Source: CAD feature listing. Evaluate the final solid. Frame: model axes, mm. Face numbers are marked on the shaded views. A direction names the side the tool comes from. Round coordinates to 2 decimals unless told otherwise and drop trailing zeros. Loops run counter-clockwise (first coordinate to the right, second up) from the corner with the lowest first, then second, coordinate; pieces in that order, holes last. Notation, with made-up numbers: (52, 51) -> (65, 51) arc R32 ccw to (65, 78) -> close; hole circle Ø7 at (-8, -15.75). An arc over 180 degrees is marked (long way). Put each result on its own line as item: value. Start each with the question number.
1. Set-up query: the marked faces 5 and 6. Return all of +Z, -Z, +X, -X, +Y, -Y with unobstructed straight access to the full face (end or side cutting, diameter ignored); none if empty.
2. Cut plane D-D (z = 2.75). Return the cut outline in (x, y) (3 decimals), then the cut area to 3 significant figures.
3. Draft query along Y for the marked faces 1, 2, 3 and 4. Return one class per face: pulls with the +Y half, pulls with the -Y half, needs draft (parallel to the pull), parting line crosses it, or undercut.
4. Cut plane C-C (x = -10). Return the cut outline in (y, z) (3 decimals), then the cut area to 3 significant figures.
5. Cut plane A-A (x = 10). Return the cut outline in (y, z) (3 decimals), then the cut area to 3 significant figures.
6. Cut plane B-B (z = 9.75). Return the cut outline in (x, y) (3 decimals).
7. Contact query for flat-ended pins moving along their axis: pin 1 (5 mm diameter, centred on y = -0.5, z = 5, fed in from +X); pin 2 (1 mm diameter, centred on y = 6, z = 10.5, fed in from -X); pin 3 (4 mm diameter, centred on y = -5, z = 8.5, fed in from +X); pin 4 (5 mm diameter, centred on x = 6.5, y = 1.5, fed in from +Z). Output: stop coordinate, or through.
8. Material intervals for L1, parallel to Y at x = 10, z = 10.3 (3 decimals); L2, parallel to Z at x = 8, y = 6.5; L3, parallel to X at y = 5.5, z = 1, sorted ascending.
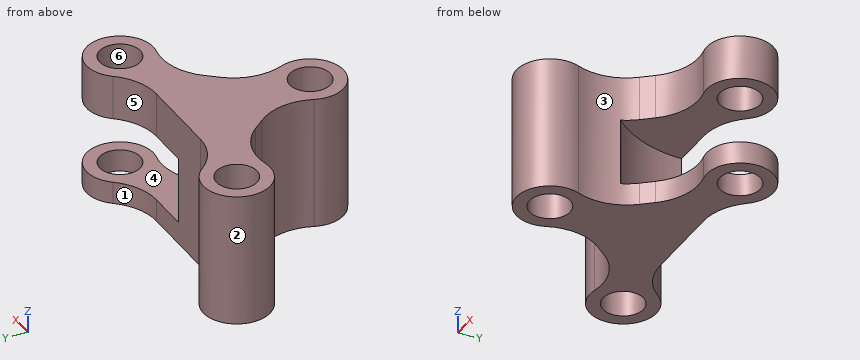
```python
from build123d import *

# Parameters (mm, degrees)
ESQUISSE2_R             = 3
ESQUISSE2_R_2           = 1.825
BOSS_EXTRU_1_DEPTH      = 12
ESQUISSE3_R             = 10
ENL_V_MAT_EXTRU_1_DEPTH = 6
CONG_1_R                = 5
FILLET1_R               = 5


with BuildPart() as part:
    # Esquisse2 → Boss.-Extru.1 (new body)
    # profile 1 of 4: a face of its own
    with BuildSketch(Plane.XY):
        with Locations((-10, 5)):
            Circle(ESQUISSE2_R)
        with Locations((-10, 5)):
            Circle(ESQUISSE2_R_2, mode=Mode.SUBTRACT)
    # profile 2 of 4: a face of its own
    with BuildSketch(Plane.XY):
        with Locations((10, 5)):
            Circle(ESQUISSE2_R)
        with Locations((10, 5)):
            Circle(ESQUISSE2_R_2, mode=Mode.SUBTRACT)
    # profile 3 of 4: a face of its own
    with BuildSketch(Plane.XY):
        with Locations((0, -6.825)):
            Circle(ESQUISSE2_R)
        with Locations((0, -6.825)):
            Circle(ESQUISSE2_R_2, mode=Mode.SUBTRACT)
    # profile 4 of 4: a face of its own
    with BuildSketch(Plane.XY):
        Polygon((-8.175, 5), (8.175, 5), (0, -5), align=None)
    extrude(amount=BOSS_EXTRU_1_DEPTH)

    # Esquisse3 → Enlèv. mat.-Extru.1 (cut)
    with BuildSketch(Plane.XY.offset(2)):
        with Locations((10, 5)):
            Circle(ESQUISSE3_R)
    extrude(amount=ENL_V_MAT_EXTRU_1_DEPTH, mode=Mode.SUBTRACT)

    # Congé1
    # the kernel refuses this fillet: 5 mm, written as the material it adds along each edge
    with BuildSketch(Plane(origin=(-7, 5, 0), x_dir=(-0.3311912213512006, 0.9435636570469954, 0), z_dir=(0, 0, 1))) as cong_1_piece_1:
        with BuildLine():
            CenterArc((3.643103435, -4.717818285), CONG_1_R, 109.341093727, 51.317812547)
            Line((-1.07471485, -3.061862178), (0, 0))
            ThreePointArc((0, 0), (0.993573664, -0.169309029), (1.987147328, 0))
        make_face()
    extrude(amount=12)
    with BuildSketch(Plane(origin=(-7.231093941, 3.845374851, 12), x_dir=(-0.7661000074497634, -0.6427213848826507, 0), z_dir=(0, 0, -1))) as cong_1_piece_2:
        with BuildLine():
            CenterArc((5.056907819, -4.440322454), CONG_1_R, 117.368969646, 63.360078756)
            Line((0.057312583, -4.503942212), (0, 0))
            ThreePointArc((0, 0), (1.379156678, -0.335806528), (2.758313356, 0))
        make_face()
    extrude(amount=12)
    with BuildSketch(Plane(origin=(-0.858096974, -3.950340093, 12), x_dir=(-0.6329215353519139, 0.7742159453846039, 0), z_dir=(0, 0, -1))) as cong_1_piece_3:
        with BuildLine():
            CenterArc((4.246739065, -5), CONG_1_R, 90, 61.27443838)
            ThreePointArc((-0.137920096, -2.596926126), (0.227062491, -1.314184518), (0, 0))
            Line((0, 0), (4.246739065, 0))
        make_face()
    extrude(amount=12)
    with BuildSketch(Plane(origin=(7.231093941, 3.845374851, 12), x_dir=(-0.6329215353519138, -0.774215945384604, 0), z_dir=(0, 0, -1))) as cong_1_piece_4:
        with BuildLine():
            CenterArc((4.504306848, -5), CONG_1_R, 90, 63.360078756)
            ThreePointArc((0.035096646, -2.758090063), (0.353327666, -1.374772245), (0, 0))
            Line((0, 0), (4.504306848, 0))
        make_face()
    extrude(amount=4)
    with BuildSketch(Plane(origin=(7, 5, 12), x_dir=(-1, 0, 0), z_dir=(0, 0, -1))) as cong_1_piece_5:
        with BuildLine():
            CenterArc((3.244997998, 5), CONG_1_R, 218.682187453, 51.317812547)
            ThreePointArc((-0.658125751, 1.875), (-0.169309029, 0.993573664), (0, 0))
            Line((0, 0), (3.244997998, 0))
        make_face()
    extrude(amount=4)
    with BuildSketch(Plane(origin=(0.858096974, -3.950340093, 12), x_dir=(0.7395598752725667, -0.6730907746261462, 0), z_dir=(0, 0, -1))) as cong_1_piece_6_section:
        with BuildLine():
            CenterArc((4.767740899, -4.505933799), CONG_1_R, 115.685497342, 61.27443838)
            Line((-0.225222573, -4.240762606), (0, 0))
            ThreePointArc((0, 0), (1.300292973, -0.29643972), (2.600585945, 0))
        make_face()
    cong_1_piece_6 = extrude(amount=12, mode=Mode.PRIVATE)
    cong_1_piece_6 = cong_1_piece_6 - Plane(origin=(10, 5, 10), x_dir=(1, 0, 0), z_dir=(0, 0, -1)) * Cylinder(10, 41, mode=Mode.PRIVATE)
    add(cong_1_piece_6)
    with BuildSketch(Plane(origin=(0.858096974, -3.950340093, 12), x_dir=(0.7395598752725667, -0.6730907746261462, 0), z_dir=(0, 0, -1))) as cong_1_piece_7_section:
        with BuildLine():
            CenterArc((4.767740899, -4.505933799), CONG_1_R, 115.685497342, 61.27443838)
            Line((-0.225222573, -4.240762606), (0, 0))
            ThreePointArc((0, 0), (1.300292973, -0.29643972), (2.600585945, 0))
        make_face()
    cong_1_piece_7 = extrude(amount=22.616847663, mode=Mode.PRIVATE)
    cong_1_piece_7 = split(cong_1_piece_7, bisect_by=Plane(origin=(2.909028405, -1.544063306, 8), z_dir=(0, 0, 1)), keep=Keep.TOP, mode=Mode.PRIVATE)
    add(cong_1_piece_7)
    with BuildSketch(Plane(origin=(0.858096974, -3.950340093, 22.616847663), x_dir=(0.7395598752725666, -0.6730907746261463, 0), z_dir=(0, 0, -1))) as cong_1_piece_8_section:
        with BuildLine():
            CenterArc((4.767740899, -4.505933799), CONG_1_R, 115.685497342, 61.27443838)
            Line((-0.225222573, -4.240762606), (0, 0))
            ThreePointArc((0, 0), (1.300292973, -0.29643972), (2.600585945, 0))
        make_face()
    cong_1_piece_8 = extrude(amount=22.616847663, mode=Mode.PRIVATE)
    cong_1_piece_8 = split(cong_1_piece_8, bisect_by=Plane(origin=(2.909028405, -1.544063306, 2), z_dir=(0, 0, -1)), keep=Keep.TOP, mode=Mode.PRIVATE)
    add(cong_1_piece_8)

    # Fillet1
    fillet1_edges = [part.edges().sort_by_distance(p)[0] for p in [
        (7.231093941, 3.845374851, 1),
        (7, 5, 1),
    ]]
    fillet(fillet1_edges, radius=FILLET1_R)


solid = part.part
```
Solution:
1. face 5: +Z, -Z, +Y
1. face 6: +Z, -Z
2. outline: (-9.344, 2.073) arc R5 cw to (-4.38, 0.358) -> (-3.546, -0.662) arc R5 cw to (-2.781, -5.701) arc R3 ccw (long way) to (2.781, -5.701) arc R5 cw to (2.791, -1.93) arc R10 cw to (0, 5) -> (-3.755, 5) arc R5 cw to (-7.658, 6.875) arc R3 ccw (long way) to start; hole circle Ø3.65 at (-10, 5); hole circle Ø3.65 at (0, -6.825)
2. area: 94.0 mm^2
3. face 1: pulls with the +Y half
3. face 2: parting line crosses it
3. face 3: undercut
3. face 4: needs draft
4. outline: (2, 0) -> (3.175, 0) -> (3.175, 12) -> (2, 12) -> close; (6.825, 0) -> (8, 0) -> (8, 12) -> (6.825, 12) -> close
4. area: 28.2 mm^2
5. outline: (2, 0) -> (3.175, 0) -> (3.175, 2) -> (2, 2) -> close; (2, 8) -> (3.175, 8) -> (3.175, 12) -> (2, 12) -> close; (6.825, 0) -> (8, 0) -> (8, 2) -> (6.825, 2) -> close; (6.825, 8) -> (8, 8) -> (8, 12) -> (6.825, 12) -> close
5. area: 14.1 mm^2
6. outline: (-9.344, 2.073) arc R5 cw to (-4.38, 0.358) -> (-3.546, -0.662) arc R5 cw to (-2.781, -5.701) arc R3 ccw (long way) to (2.781, -5.701) arc R5 cw to (3.546, -0.662) -> (4.38, 0.358) arc R5 cw to (9.344, 2.073) arc R3 ccw (long way) to (7.658, 6.875) arc R5 cw to (3.755, 5) -> (-3.755, 5) arc R5 cw to (-7.658, 6.875) arc R3 ccw (long way) to start; hole circle Ø3.65 at (-10, 5); hole circle Ø3.65 at (0, -6.825); hole circle Ø3.65 at (10, 5)
7. pin 1: stops at x = 2.79
7. pin 2: stops at x = -12.96
7. pin 3: stops at x = 3
7. pin 4: stops at z = 12
8. L1: y = 2 to 3.175, 6.825 to 8
8. L2: z = 0 to 2, 8 to 12
8. L3: x = -12.96 to -11.76, -8.24 to -5.93, 5.93 to 8.24, 11.76 to 12.96
